Part model, mm, in its own coordinate system. Face numbers are marked on the shaded views. A direction names the side the tool comes from. Coordinates: 2 decimals unless noted, no trailing zeros. Write each loop counter-clockwise with the first axis right and the second up, starting at its lowest first coordinate (ties: lowest second). Pieces come first, ordered by that corner, then holes. Notation, with made-up numbers: (2, -24.5) -> (24, -24.5) arc R22 cw to (24, 11.5) -> close; hole circle Ø2 at (32, 86.5). An arc over 180 degrees is marked (long way). One line per question, with ' | ' between items. Start each with the question number.
Item 1: Saw through at A-A (y = -0.5). List the corners of the cut face in (x, z), and give its area (3 significant figures).
Item 2: Saw through at B-B (x = 82.5). List the corners of the cut face in (y, z).
Item 3: Saw through at C-C (y = 27). List the corners of the cut face in (x, z), and give its area (3 significant figures).
Item 4: Probe probe 1 along X at (y, z) = (11.5, 329); probe 2 along Z at (x, y) = (86, 37); probe 3 along Y at (x, z) = (-2.5, 122). List the from-to ranges inside material, lowest first. Write a range as [from, to].
Item 5: 3-axis set-ups, long thin cutter, end or side, ignore diameter. For the marked faces 1 and 2: which of +Z, -Z, +X, -X, +Y, -Y reach the whole face in a straight line?
Item 6: Pin check, flat tips, straight feed: pin 1 (5 mm diameter, centred on y = 16, z = 244, fed in from +X); pin 2 (1.5 mm diameter, centred on x = 32, y = 40.5, fed in from +Z); pin 3 (1 mm diameter, centred on y = 3, z = 345, fed in from +X). Stop position of each tip, or through.
Item 7: Saw through at D-D (z = 218.5). List the corners of the cut face in (x, y).
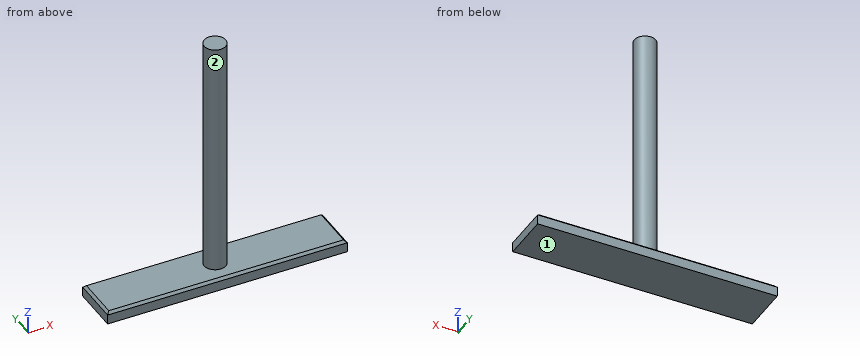
from build123d import *

# Parameters (mm, degrees)
F0_R     = 22.5
F1_DEPTH = 500
F2_W     = 500
F2_H     = 100
F3_DEPTH = 25.4
F4_SIZE  = 5.08


with BuildPart() as f1:
    # F0 (on Top) → F1 (new body)
    with BuildSketch(Plane.XY):
        with Locations((-2.513092, 12.474374)):
            Circle(F0_R)
    extrude(amount=F1_DEPTH)

    # F2 (on face) → F3 (join)
    with BuildSketch(Plane(origin=(0, 0, 0), x_dir=(1, 0, 0), z_dir=(0, 0, -1))):
        with Locations((-2.513092, -12.474374)):
            Rectangle(F2_W, F2_H)
    extrude(amount=F3_DEPTH)

    # F4
    f4_edges = [f1.edges().sort_by_distance(p)[0] for p in [
        (-2.513092, -37.525626, 0),
        (-252.513092, 12.474374, 0),
        (-2.513092, 62.474374, 0),
        (247.486908, 12.474374, 0),
    ]]
    chamfer(f4_edges, length=F4_SIZE)


solid = f1.part
From the geometry:
1) outline: (-252.51, -25.4) -> (247.49, -25.4) -> (247.49, -5.08) -> (242.41, 0) -> (15.87, 0) -> (15.87, 500) -> (-20.9, 500) -> (-20.9, 0) -> (-247.43, 0) -> (-252.51, -5.08) -> close | area: 31,100 mm2
2) outline: (-37.53, -25.4) -> (62.47, -25.4) -> (62.47, -5.08) -> (57.39, 0) -> (-32.45, 0) -> (-37.53, -5.08) -> close
3) outline: (-252.51, -25.4) -> (247.49, -25.4) -> (247.49, -5.08) -> (242.41, 0) -> (14.67, 0) -> (14.67, 500) -> (-19.7, 500) -> (-19.7, 0) -> (-247.43, 0) -> (-252.51, -5.08) -> close | area: 29,900 mm2
4) probe 1: [-24.99, 19.97] | probe 2: [-25.4, 0] | probe 3: [-10.03, 34.97]
5) face 1: -Z, +X, -X, +Y, -Y | face 2: +Z
6) pin 1: x = 19.96 | pin 2: z = 0 | pin 3: x = 18.12
7) outline: circle Ø45 at (-2.51, 12.47)
